```python
from build123d import *

# Parameters (mm, degrees)
BOSS_EXTRUDE1_DEPTH = 40
SKETCH4_R           = 4.5
SKETCH4_R_2         = 2.1
BOSS_EXTRUDE4_DEPTH = 10
FILLET2_R           = 1
SKETCH5_R           = 2
CUT_EXTRUDE1_DEPTH  = 44.543082261


with BuildPart() as part:
    # Sketch1 → Boss-Extrude1 (new body)
    with BuildSketch(Plane.XY):
        Polygon((-11, 3.3), (-11, 5), (4, 5), (4, -5), (-11, -5), (-11, 0), (0, 0), (0, 3.3), align=None)
    extrude(amount=BOSS_EXTRUDE1_DEPTH)

    # Sketch4 → Boss-Extrude4 (add)
    with BuildSketch(Plane(origin=(4, 0, 0), x_dir=(0, 0, -1), z_dir=(1, 0, 0))):
        with Locations(Location((-20, 0, 0), (0, 0, 90))):
            Circle(SKETCH4_R)
        with Locations(Location((-20, 0, 0), (0, 0, 90))):
            Circle(SKETCH4_R_2, mode=Mode.SUBTRACT)
    extrude(amount=BOSS_EXTRUDE4_DEPTH)

    # Fillet2
    fillet2_edges = [part.edges().sort_by_distance(p)[0] for p in [
        (4, -4.5, 20),
    ]]
    fillet(fillet2_edges, radius=FILLET2_R)

    # Sketch5 → Cut-Extrude1 (cut, through all)
    with BuildSketch(Plane(origin=(0, 5, 0), x_dir=(1, 0, 0), z_dir=(0, 1, 0))):
        with Locations(Location((-8, -36, 0), (0, 0, 270))):
            Circle(SKETCH5_R)
        with Locations(Location((-8, -4, 0), (0, 0, 270))):
            Circle(SKETCH5_R)
    extrude(amount=-CUT_EXTRUDE1_DEPTH, mode=Mode.SUBTRACT)


solid = part.part
```
Read the model definition and answer for the solid it produces. Units are mm, in the model's axes. A direction names the side the tool comes from. Give positions to 0.01 mm unless a question says otherwise; leave off trailing zeros. Loops run counter-clockwise (first coordinate to the right, second up) from the corner with the lowest first, then second, coordinate; pieces in that order, holes last.
Item 1: Find the intervals of material crossed by line 1 along Y through (x, z) = (-8.5, 33); line 2 along X through (y, z) = (3.7, 4); line 3 along Z through (x, y) = (9.5, 0), in increasing order.
Item 2: The part is cut by section A-A (x = -8). Write down the section's boundary in (y, z).
Item 3: For faces 1 (the cylindrical face through (-6.648, -2.465, 2.526)), 2 (the flat face through (-5, 3.3, 20)), 3 (the cylindrical face through (8.93, 1.13, 21.77)), determine the directions among +Z, -Z, +X, -X, +Y, -Y from which every point of the face is accessible in a straight line to the end or side of a thin tool.
Item 4: Each of these flat-tipped pins is pushed along its axis until it touches: pin 1 Ø4.5 at (y, z) = (0, 19.5) entering from +X; pin 2 Ø1.5 at (x, y) = (8, -2.5) entering from -Z; pin 3 Ø3 at (y, z) = (2.5, 32.5) entering from +X; pin 4 Ø3 at (x, z) = (7, 25.5) entering from +Y. Where does it stop, or does it pass through?
Item 5: The part is cut by section B-B (z = 4). Write down the section's boundary in (x, y).
Item 6: The part is cut by section D-D (z = 27). Write down the section's boundary in (x, y), and give its area (3 significant figures).
Item 7: The part is cut by section C-C (x = -2.5). Write down the section's boundary in (y, z), and give its area (3 significant figures).
Item 8: The mould has two halves that part along Y. Classify faces 4 (the flat face through (4, 0, 20)), 5 (the flat face through (-4, 5, 20)), 6 (the flat face through (-6, 0, 20)), 7 (the flat face through (4, 0, 7)): released by +Y, released by -Y, zero draft, split by the parting line, or undercut.
Taken from the geometry:
1. line 1: y = -5 to 0, 3.3 to 5
1. line 2: x = -11 to -10, -6 to 4
1. line 3: z = 15.5 to 17.9, 22.1 to 24.5
2. outline: (-5, 0) - (0, 0) - (0, 2) - (-5, 2) - close; (-5, 6) - (0, 6) - (0, 34) - (-5, 34) - close; (-5, 38) - (0, 38) - (0, 40) - (-5, 40) - close; (3.3, 0) - (5, 0) - (5, 2) - (3.3, 2) - close; (3.3, 6) - (5, 6) - (5, 34) - (3.3, 34) - close; (3.3, 38) - (5, 38) - (5, 40) - (3.3, 40) - close
3. face 1: +Y, -Y
3. face 2: +Z, -Z, -X
3. face 3: +X
4. pin 1: stops at x = 14
4. pin 2: stops at z = 15.85
4. pin 3: stops at x = 4
4. pin 4: stops at y = 2.06
5. outline: (-11, -5) - (-10, -5) - (-10, 0) - (-11, 0) - close; (-11, 3.3) - (-10, 3.3) - (-10, 5) - (-11, 5) - close; (-6, -5) - (4, -5) - (4, 5) - (-6, 5) - (-6, 3.3) - (0, 3.3) - (0, 0) - (-6, 0) - close
6. outline: (-11, -5) - (4, -5) - (4, 5) - (-11, 5) - (-11, 3.3) - (0, 3.3) - (0, 0) - (-11, 0) - close
6. area: 114 mm2
7. outline: (-5, 0) - (0, 0) - (0, 40) - (-5, 40) - close; (3.3, 0) - (5, 0) - (5, 40) - (3.3, 40) - close
7. area: 268 mm2
8. face 4: undercut
8. face 5: released by +Y
8. face 6: undercut
8. face 7: zero draft
